Can you work these out from the model? Positions are in its coordinate system, mm. Round coordinates to 2 decimals unless told otherwise and drop trailing zeros. Use CSV: the item, a comma, the result in double quotes.
Autodesk Inventor part; units mm, degrees
ref_plane "YZ Plane" through (0, 0, 0) normal (1, 0, 0) x (0, 1, 0)
ref_plane "XZ Plane" through (0, 0, 0) normal (0, 1, 0) x (-1, 0, 0)
ref_plane "XY Plane" through (0, 0, 0) normal (0, 0, 1) x (1, 0, 0)
sketch "Skizze1" plane through (0, 0, 0) normal (0, 0, 1) x (1, 0, 0)
  line L0 (-1.2, 0) -> (7.2, 0)
  line L1 (0, -2) -> (0, 12)
  line L2 (0, 7) -> (0, 2.3098)
  line L3 (0, 2.3098) -> (1.5, 0)
  line L4 (1.5, 0) -> (4.5, 0)
  line L5 (4.5, 0) -> (6, 2.3098)
  line L6 (6, 2.3098) -> (6, 7)
  arc A0 (6, 7) -> (0, 7) centre (3, 7) ccw
  point P0 (0, 0)
  dimension "d0" = 33
  dimension "d1" = 33
  dimension "d2" = 3
  dimension "d3" = 10
  dimension "d4" = 1.5
  dimension "d5" = 3
extrude "Extrusion1" add sketch "Skizze1" along normal mid plane 4 contours L3 L1 A0 L6 L5 L0
sketch "Skizze2" plane through (0, 0, -2) normal (0, 0, -1) x (-1, 0, 0)
  arc A0 (0, 7) -> (-6, 7) centre (-3, 7) ccw
  point P0 (0, 0)
hole "Bohrung1" at (3, 7, -2) at (3, 7, -2) direction (0, 0, 1) diameter 4 end through all
sketch "Skizze3" plane through (1.5, 0, 2) normal (0, -1, 0) x (1, 0, 0)
  line L0 (-2.7, -2) -> (5.7, -2)
  line L1 (-1.5, -4.8) -> (-1.5, 0.8)
  point P0 (-1.5, -2)
  point P1 (1.5, -2)
  dimension "d15" = 3
hole "Bohrung2" at (3, 0, 0) direction (0, 1, 0) diameter 2.459 depth 4 tip angle 118
sketch "Skizze4" plane through (1.5, 0, 2) normal (0, -1, 0) x (1, 0, 0)
  arc A0 (3.7361, -4) -> (3.7361, 0) centre (1.5, -2) ccw
  line L0 (3.7361, 0) -> (5.5, 0)
  line L1 (5.5, 0) -> (5.5, -4)
  line L2 (5.5, -4) -> (3.7361, -4)
  line L3 (4.5, -4) -> (3, -4)
  line L4 (3, 0) -> (4.5, 0)
  line L5 (4.5, -4) -> (4.5, 0)
  dimension "d24" = 3
  dimension "d25" = 4
sketch "Skizze5" plane through (0, 0, 2) normal (0, 0, 1) x (1, 0, 0)
  line L0 (6, 0) -> (6, 7)
  line L1 (6, 2.3098) -> (6, 7)
  arc A0 (6, 7) -> (0, 7) centre (3, 7) ccw
  line L2 (0, 7) -> (0, 2.3098)
  arc A1 (6, 7) -> (0, 7) centre (3, 7) ccw
  line L3 (0, 7) -> (0, 0)
sweep "Sweeping2" cut profiles "Skizze4" path "Skizze5" path curves L0 A1 L3
chamfer "Fase2" distance 0.5 angle 45 2 edges at (3, 0, 2) (3, 0, -2)
properties part number "Pleuelkopf"
Q1. Will these pins go through, and if not, where does the flat tip stop? P1, Ø1, axis at x = 0.5, z = -0.5, coming from the -Y side; P2, Ø1, axis at y = 1.5, z = 1, coming from the -X side.
Resolved:
P1,"stops at y = 0.77"
P2,"stops at x = 0.2"
Q2. If we mould it in two halves opening along X, with no side actions, what happens to faces 1 (the face through (5.795, 4.76, 1.09)), 2 (the face through (0.205, 4.678, 1.09)), 3 (the face through (1.78, 2.03, 0.16))? For each: released by +X, released by -X, zero draft, split by the parting line, or undercut.
Resolved:
face 1,"released by +X"
face 2,"released by -X"
face 3,"undercut"
Q3. Please list where these lines run through material, in increasing order: probe 1 along Z at (x, y) = (3, 2.15); probe 2 along Y at (x, z) = (2.25, 0.05); probe 3 along Y at (x, z) = (2.75, 0.95).
Resolved:
probe 1,"z = -2 to -1.23, 1.23 to 2"
probe 2,"y = 4.29 to 5.15, 8.85 to 9.9"
probe 3,"y = 4.15 to 5.02, 8.98 to 9.83"
